Autodesk Inventor part; units mm, degrees
ref_plane "YZ Plane" through (0, 0, 0) normal (1, 0, 0) x (0, 1, 0)
ref_plane "XZ Plane" through (0, 0, 0) normal (0, 1, 0) x (-1, 0, 0)
ref_plane "XY Plane" through (0, 0, 0) normal (0, 0, 1) x (1, 0, 0)
sketch "Sketch1" plane through (0, 0, 0) normal (0, 0, 1) x (1, 0, 0)
  line L0 (-100, 0) -> (1200, 0)
  line L1 (-100, 0) -> (-100, 16.7)
  line L2 (100, 0) -> (100, 16.15)
  line L3 (200, 0) -> (200, 15.15)
  line L4 (300, 0) -> (300, 14.2)
  line L5 (400, 0) -> (400, 13.69)
  line L6 (500, 0) -> (500, 13.5)
  line L7 (600, 0) -> (600, 13.29)
  line L8 (700, 0) -> (700, 13.175)
  line L9 (800, 0) -> (800, 12.95)
  line L10 (900, 0) -> (900, 12.9)
  line L11 (1000, 0) -> (1000, 12.85)
  line L12 (1100, 0) -> (1100, 12.4)
  line L13 (1200, 0) -> (1200, 12.4)
  line L14 (1200, 0) -> (1200, 11.25)
  line L15 (-100, 16.7) -> (100, 16.15)
  line L16 (100, 16.15) -> (200, 15.15)
  line L17 (200, 15.15) -> (300, 14.2)
  line L18 (300, 14.2) -> (400, 13.69)
  line L19 (400, 13.69) -> (500, 13.5)
  line L20 (500, 13.5) -> (600, 13.29)
  line L21 (600, 13.29) -> (700, 13.175)
  line L22 (700, 13.175) -> (800, 12.95)
  line L23 (800, 12.95) -> (900, 12.9)
  line L24 (900, 12.9) -> (1000, 12.85)
  line L25 (1000, 12.85) -> (1100, 12.4)
  line L26 (1100, 12.4) -> (1200, 12.4)
  line L27 (1200, 12.4) -> (1200, 11.25)
  point P0 (0, 0)
  point P1 (1100, 12.3857)
  point P2 (1090, 12.3713)
  point P3 (1080, 12.357)
  point P4 (1070, 12.3426)
  point P5 (1060, 12.3283)
  point P6 (1050, 12.3139)
  point P7 (1010, 11.54)
  point P8 (1020, 11.7067)
  point P9 (1030, 12.2852)
  point P10 (1040, 12.2996)
  dimension "d0" = 1300
  dimension "d1" = 100
  dimension "d2" = 100
  dimension "d3" = 100
  dimension "d4" = 100
  dimension "d5" = 100
  dimension "d6" = 100
  dimension "d7" = 100
  dimension "d8" = 100
  dimension "d9" = 100
  dimension "d10" = 100
  dimension "d11" = 100
  dimension "d12" = 100
  dimension "d13" = 16.7
  dimension "d14" = 16.15
  dimension "d15" = 15.15
  dimension "d16" = 14.2
  dimension "d17" = 13.69
  dimension "d18" = 13.5
  dimension "d19" = 13.29
  dimension "d20" = 13.175
  dimension "d21" = 12.95
  dimension "d22" = 12.9
  dimension "d23" = 12.85
  dimension "d24" = 12.4
  dimension "d25" = 12.4
  dimension "d26" = 11.25
  dimension "d31" = 100
revolve "Revolution4" add sketch "Sketch1" angle 360 about axis through (-100, 0, 0) along (1, 0, 0)
properties part number "1P.02.01.02-RN-MainSpar" material "CFRP"
The model under review builds one solid part; all positions refer to its coordinate system, in mm. A direction names the side the tool comes from. Coordinates: 2 decimals unless noted, no trailing zeros. Loops run counter-clockwise (first coordinate to the right, second up) from the corner with the lowest first, then second, coordinate; pieces in that order, holes last. Notation, with made-up numbers: M 41,66 L 74,66 A21 ccw 74,92 Z; hole C -21,11.5 d7. An arc over 180 degrees is marked long. Put each result on its own line as item: value. Start each with the question number.
Q1. Add section A-A (x = 432). Write out the cut boundary in (y, z).
Q2. Wall thickness on line 1 (Z direction, x = 95.5, y = 9); line 2 (Y direction, x = 217.5, z = 8); line 3 (Y direction, x = 1044, z = 2.5): over which ranges is each line inside the solid? List them lowest first.
Q3. For faces 1 (the cylindrical face through (1150.7, 5.72, -11)), 2 (the flat face through (1200, 0, 0)), list the 3-axis set-ups (+Z, -Z, +X, -X, +Y, -Y) from which the entire face can be reached by the end or side of a thin tool; tool diameter is ignored.
Q4. Clearance check with flat-ended pins moving along their axes: pin 1 (10 mm diameter, centred on x = 571, y = 8, fed in from +Z); pin 2 (1 mm diameter, centred on x = 868, y = 2.5, fed in from -Z); pin 3 (10 mm diameter, centred on x = 114.5, z = -4.5, fed in from +Y). State where each tip first meets the part, or that it passes through.
Q5. Add section B-B (x = -19.5). Write out the cut boundary in (y, z).
Answers:
1. outline: C 0,0 d27.26
2. line 1: z = -13.42 to 13.42
2. line 2: y = -12.67 to 12.67
2. line 3: y = -12.4 to 12.4
3. face 1: +X
3. face 2: +Z, -Z, +X, +Y, -Y
4. pin 1: stops at z = 13.01
4. pin 2: stops at z = -12.76
4. pin 3: stops at y = 16.03
5. outline: C 0,0 d32.96
